CAD build for the part. Positions are in the model's coordinates, mm. Face numbers are marked on the shaded views. A direction names the side the tool comes from. Coordinates: 2 decimals unless noted, no trailing zeros. Order: outer loops, then holes, each group sorted by start corner. A loop starts at its lowest first (then second) coordinate and runs counter-clockwise, first axis right, second up. Notation, with made-up numbers: M 88,15.25 L 98,15.25 A23 cw 98,28.25 Z; hole C 57,72 d2. An arc over 180 degrees is marked long. Write item = value, one per line.
from build123d import *

# Parameters (mm, degrees)
F1_DEPTH  = 2
F3_DEPTH  = 60
F5_DEPTH  = 31.001
F6_R      = 1.75
F7_DEPTH  = 2.001
F9_R      = 1.75
F10_DEPTH = 2.001
F13_DEPTH = 71.5924333795
F14_SIZE  = 1.2


with BuildPart() as f1:
    # F0 (on Top) → F1 (new body)
    with BuildSketch(Plane.XY):
        Polygon((62, 0), (31, 31), (0, 0), align=None)
    extrude(amount=F1_DEPTH)

    # F2 (on face) → F3 (join)
    with BuildSketch(Plane.XY.offset(2)):
        Polygon((2, 2), (0, 0), (62, 0), (60, 2), align=None)
    extrude(amount=F3_DEPTH)

    # F4 (on face) → F5 (cut, through all)
    with BuildSketch(Plane.XZ):
        Polygon((62, 62), (0, 62), (62, 0), align=None)
    extrude(amount=-F5_DEPTH, mode=Mode.SUBTRACT)

    # F6 (on face) → F7 (cut, through all)
    with BuildSketch(Plane(origin=(0, 2, 0), x_dir=(-1, 0, 0), z_dir=(0, 1, 0))):
        with Locations((-14.75, 14.75)):
            Circle(F6_R)
        with Locations((-14.75, 37.704058454)):
            Circle(F6_R)
        with Locations((-37.704058454, 14.75)):
            Circle(F6_R)
    extrude(amount=-F7_DEPTH, mode=Mode.SUBTRACT)

    # F8: F1 across face


with BuildPart() as f1_1:
    add(f1.part)
    add(f1.part.mirror(Plane(origin=(5.9907407407, 5.9907407407, 20.9962962963), x_dir=(-0.7071067812, -0.7071067812, 0), z_dir=(-0.7071067812, 0.7071067812, 0))))

    # F9 (on face) → F10 (cut, through all)
    with BuildSketch(Plane.XY.offset(2)):
        with Locations((14.75, 14.75)):
            Circle(F9_R)
        with Locations((37.704058454, 14.75)):
            Circle(F9_R)
        with Locations((14.75, 37.704058454)):
            Circle(F9_R)
    extrude(amount=-F10_DEPTH, mode=Mode.SUBTRACT)

    # F12 (on 3pt) → F13 (cut, through all)
    with BuildSketch(Plane(origin=(20.6666666667, 20.6666666667, 20.6666666667), x_dir=(0.8164965809, -0.4082482905, -0.4082482905), z_dir=(-0.5773502692, -0.5773502692, -0.5773502692))):
        Polygon((-25.3113940088, -43.8406204336), (50.6227880175, 0), (-25.3113940088, 43.8406204336), align=None)
    extrude(amount=-F13_DEPTH, mode=Mode.SUBTRACT)

    # F14
    f14_edges = [f1_1.edges().sort_by_distance(p)[0] for p in [
        (13, 37.704058, 0),
        (13, 14.75, 0),
        (35.954058, 14.75, 0),
        (0, 16.5, 14.75),
        (0, 39.454058, 14.75),
        (0, 16.5, 37.704058),
        (16.5, 0, 37.704058),
        (39.454058, 0, 14.75),
        (16.5, 0, 14.75),
    ]]
    chamfer(f14_edges, length=F14_SIZE)


solid = f1_1.part
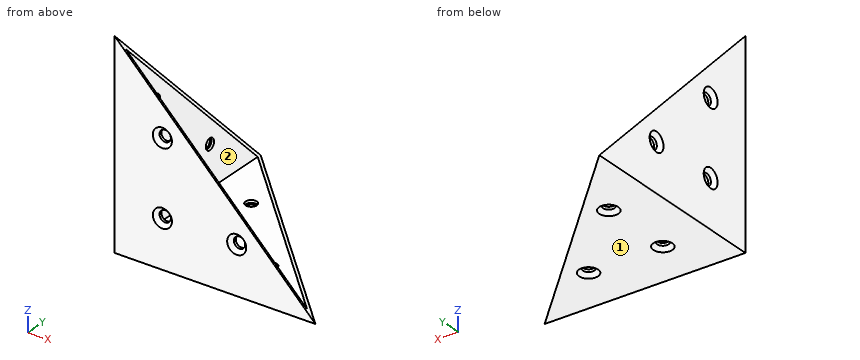
(1) Tool access for the marked faces 1 and 2: list every direction of +Z, -Z, +X, -X, +Y, -Y with a clear straight run to the whole face (end or side of a thin tool).
Evaluation:
face_1 = -Z, +X, -X, +Y, -Y
face_2 = +Z, +X, +Y
(2) Wall check: line 1 (Z direction, x = 1, y = 14); line 2 (X direction, y = 15, z = 24); line 3 (Y direction, x = 14.75, z = 1.75). Give the ranges that are in metal, low to high. Write a range as from..to.
Evaluation:
line_1 = 0..12.95, 16.55..35.9, 39.5..47
line_2 = 0..2
line_3 = 0..13, 16.5..35.95, 39.45..45.5
(3) Slice it at A-A, the plane y = 14.75. State how many separate pieces and enclosed holes the cut face has, then the cut area to 3 significant figures.
Evaluation:
separate_pieces = 5
enclosed_holes = 0
area = 147 mm²
(4) Slice it at D-D, the plane y = 4.5. Write the cut outline in (x, z).
Evaluation:
outline = M 0,0 L 57.5,0 L 55.5,2 L 2,2 L 2,55.5 L 0,57.5 Z
(5) Slice it at C-C, the plane z = 47.5. Write the cut outline in (x, y), then the cut area to 3 significant figures.
Evaluation:
outline = M 0,0 L 14.5,0 L 12.5,2 L 2,2 L 2,12.5 L 0,14.5 Z
area = 50.0 mm²
(6) Pin check, flat tips, straight feed: pin 1 Ø5.5 at (x, y) = (14.75, 37.7) entering from +Z; pin 2 Ø10 at (x, z) = (29, 39.5) entering from +Y; pin 3 Ø3 at (x, y) = (14.75, 14.75) entering from +Z; pin 4 Ø4.5 at (x, z) = (14.75, 37.7) entering from -Y. Stop position of each tip, or through.
Evaluation:
pin_1 = 2
pin_2 = 0.57
pin_3 = through
pin_4 = 0.7
